Could you check a few things on this drawing? It's one solid part, dimensions in mm from its lowest x, y, z. Coordinates: 2 decimals unless noted, no trailing zeros. Write each loop counter-clockwise with the first axis right and the second up, starting at its lowest first coordinate (ties: lowest second). Pieces come first, ordered by that corner, then holes. Notation, with made-up numbers: (43, -28.75) - (57, -28.75) arc R17 cw to (57, -9.75) - close; hole circle Ø10 at (10.5, -33.75). An arc over 180 degrees is marked (long way). Use one line per item in the form item = value. Start each with the question number.
(1) For pin 1 Ø4.5 at (x, y) = (6.35, 31.75) entering from +Z, with a flat end and sliding along its axis, tell me the tip position at first contact or that it passes through.
(2) If I drill on probe 1 along Y at (x, z) = (6.35, 0.7); probe 2 along X at (y, z) = (31.75, 1.25); probe 3 along Y at (x, z) = (7, 1.4) (1 decimal), over which ranges is the centre line in solid material (lowest first)? Write a range as from..to.
(3) If we section it at A-A on z = 1: Give the number of separate pieces and of enclosed holes in the cut face, then the cut area to 3 significant figures.
(4) If we section it at B-B on y = 6.35: Please give me the cut outline in (x, z), then the cut area to 3 significant figures.
(5) If we section it at C-C on x = 6.35: Please give me the cut outline in (y, z).
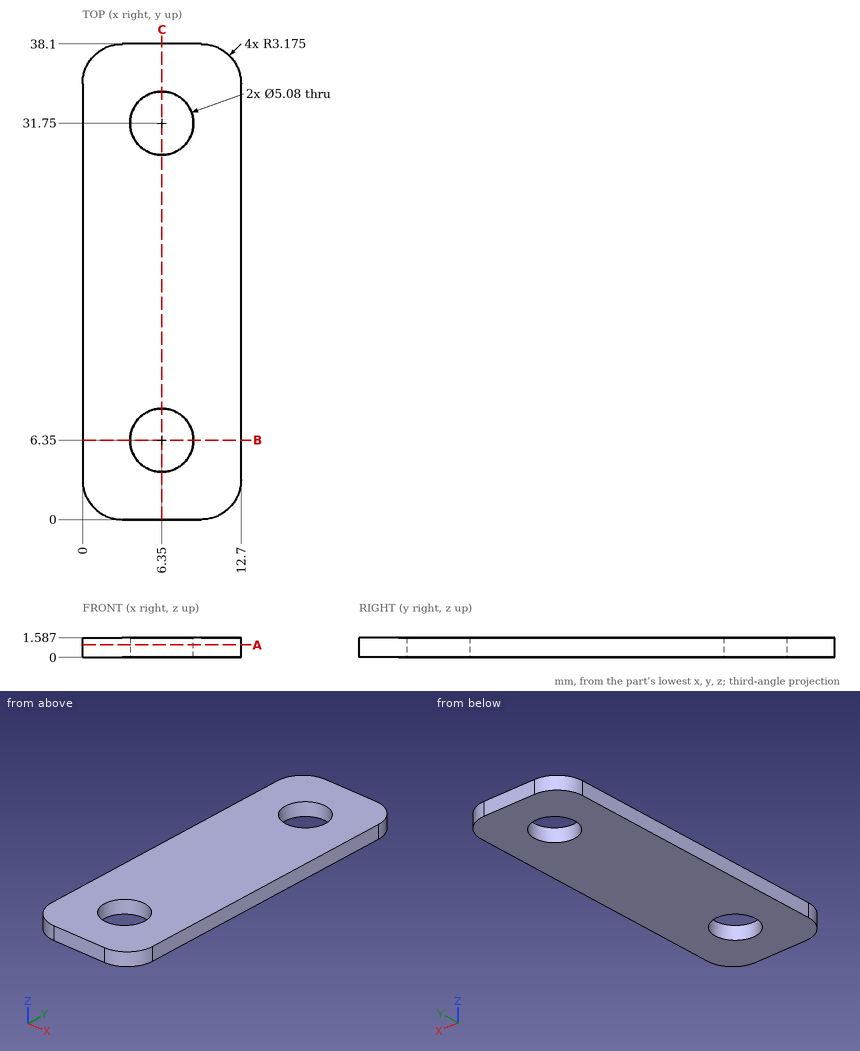
Reported:
q1.pin_1 = through
q2.probe_1 = 0..3.81, 8.89..29.21, 34.29..38.1
q2.probe_2 = 0..3.81, 8.89..12.7
q2.probe_3 = 0..3.9, 8.8..29.3, 34.2..38.1
q3.separate_pieces = 1
q3.enclosed_holes = 2
q3.area = 435 mm2
q4.outline = (0, 0) - (3.81, 0) - (3.81, 1.59) - (0, 1.59) - close; (8.89, 0) - (12.7, 0) - (12.7, 1.59) - (8.89, 1.59) - close
q4.area = 12.1 mm2
q5.outline = (0, 0) - (3.81, 0) - (3.81, 1.59) - (0, 1.59) - close; (8.89, 0) - (29.21, 0) - (29.21, 1.59) - (8.89, 1.59) - close; (34.29, 0) - (38.1, 0) - (38.1, 1.59) - (34.29, 1.59) - close
